Part model, mm, in its own coordinate system. A direction names the side the tool comes from. Give positions to 0.01 mm unless a question says otherwise; leave off trailing zeros. Loops run counter-clockwise (first coordinate to the right, second up) from the corner with the lowest first, then second, coordinate; pieces in that order, holes last. Notation, with made-up numbers: M 64,28.5 L 120,28.5 A29 cw 120,54.5 Z; hole C -7,29 d4. An arc over 180 degrees is marked long. Answer in a Markdown table with one row per item.
from build123d import *

# Parameters (mm, degrees)
SKETCH_1_W               = 58
SKETCH_1_H               = 44
SKETCH_1_R               = 1.6
EXTRUDE_1_DEPTH          = 1
SKETCH_2_W               = 132.5
SKETCH_2_H               = 90
EXTRUDE_2_DEPTH          = 1
SKETCH_6_W               = 15
SKETCH_6_H               = 90
CUT_EXTRUDE_4_DEPTH      = 1
CUT_EXTRUDE_4_DEPTH_BACK = 2
CUT_EXTRUDE_6_DEPTH      = 2
EXTRUDE_3_DEPTH          = 1
EXTRUDE_4_DEPTH          = 1
SKETCH_11_R              = 1.6
CUT_EXTRUDE_7_DEPTH      = 2
CUT_EXTRUDE_8_DEPTH      = 2
FILLET_3_R               = 2
SKETCH_14_R              = 1.6
CUT_EXTRUDE_9_DEPTH      = 2
SKETCH_15_R              = 9
CUT_EXTRUDE_10_DEPTH     = 2
CUT_EXTRUDE_11_DEPTH     = 2


with BuildPart() as part:
    # 草图1 → 凸台-拉伸1 (new body)
    with BuildSketch(Plane(origin=(0, 0, 0), x_dir=(0, 0, -1), z_dir=(1, 0, 0))):
        with Locations((19, -14.5)):
            Rectangle(SKETCH_1_W, SKETCH_1_H)
        Circle(SKETCH_1_R, mode=Mode.SUBTRACT)
        with Locations((17, 0)):
            Circle(SKETCH_1_R, mode=Mode.SUBTRACT)
        with Locations((0, -30.5)):
            Circle(SKETCH_1_R, mode=Mode.SUBTRACT)
        with Locations((17, -30.5)):
            Circle(SKETCH_1_R, mode=Mode.SUBTRACT)
        with Locations((31.5, -30.5)):
            Circle(SKETCH_1_R, mode=Mode.SUBTRACT)
    extrude(amount=EXTRUDE_1_DEPTH)

    # 草图2 → 凸台-拉伸2 (add)
    with BuildSketch(Plane(origin=(1, 0, 0), x_dir=(0, 0, -1), z_dir=(1, 0, 0))):
        with Locations((-18.25, 52.5)):
            Rectangle(SKETCH_2_W, SKETCH_2_H)
    extrude(amount=-EXTRUDE_2_DEPTH)

    # 草图6 → 切除-拉伸4 (cut, two sides)
    with BuildSketch(Plane(origin=(1, 0, 0), x_dir=(0, 0, -1), z_dir=(1, 0, 0))) as cut_extrude_4_sk:
        with Locations((40.5, 52.5)):
            Rectangle(SKETCH_6_W, SKETCH_6_H)
    extrude(amount=CUT_EXTRUDE_4_DEPTH, mode=Mode.SUBTRACT)
    extrude(cut_extrude_4_sk.sketch, amount=-CUT_EXTRUDE_4_DEPTH_BACK, mode=Mode.SUBTRACT)

    # 草图8 → 切除-拉伸6 (cut, through all)
    with BuildSketch(Plane(origin=(1, 0, 0), x_dir=(0, 0, -1), z_dir=(1, 0, 0))):
        Polygon((-84.5, 7.5), (-10, 7.5), (-10, 6.5), (48, 6.5), (48, 7.5), (33, 7.5), (33, 97.5), (-84.5, 97.5), align=None)
    extrude(amount=-CUT_EXTRUDE_6_DEPTH, mode=Mode.SUBTRACT)

    # 草图9 → 凸台-拉伸3 (add)
    with BuildSketch(Plane(origin=(1, 0, 0), x_dir=(0, 0, -1), z_dir=(1, 0, 0))):
        Polygon((-10, -32.5), (-10, 3.4), (-85.916522377, 1.4), (-95, -32.5), (-10, -36.5), align=None)
    extrude(amount=-EXTRUDE_3_DEPTH)

    # 草图10 → 凸台-拉伸4 (add)
    with BuildSketch(Plane(origin=(1, 0, 0), x_dir=(0, 0, -1), z_dir=(1, 0, 0))):
        Polygon((40.4, -45.5), (58.4, -45.5), (58.4, 6.5), (48, 6.5), (48, -36.5), (40.4, -36.5), align=None)
    extrude(amount=-EXTRUDE_4_DEPTH)

    # 草图11 → 切除-拉伸7 (cut, through all)
    with BuildSketch(Plane(origin=(1, 0, 0), x_dir=(0, 0, -1), z_dir=(1, 0, 0))):
        with Locations((45.4, -42.5)):
            Circle(SKETCH_11_R)
        with Locations((53.4, -42.5)):
            Circle(SKETCH_11_R)
    extrude(amount=-CUT_EXTRUDE_7_DEPTH, mode=Mode.SUBTRACT)

    # 草图13 → 切除-拉伸8 (cut, through all)
    with BuildSketch(Plane(origin=(1, 0, 0), x_dir=(0, 0, -1), z_dir=(1, 0, 0))):
        Polygon((24.2, 6.5), (58.4, -19.5), (58.4, 6.5), align=None)
    extrude(amount=-CUT_EXTRUDE_8_DEPTH, mode=Mode.SUBTRACT)

    # 圆角3
    fillet_3_edges = [part.edges().sort_by_distance(p)[0] for p in [
        (0.5, -32.5, 95),
        (0.5, 1.4, 85.916522377),
        (0.5, -45.5, -58.4),
        (0.5, -45.5, -40.4),
        (0.5, -36.5, -40.4),
        (0.5, 6.5, -24.2),
        (0.5, -19.5, -58.4),
    ]]
    fillet(fillet_3_edges, radius=FILLET_3_R)

    # 草图14 → 切除-拉伸9 (cut, through all)
    with BuildSketch(Plane(origin=(1, 0, 0), x_dir=(0, 0, -1), z_dir=(1, 0, 0))):
        with Locations((55.5, -30.5)):
            Circle(SKETCH_14_R)
    extrude(amount=-CUT_EXTRUDE_9_DEPTH, mode=Mode.SUBTRACT)

    # 草图15 → 切除-拉伸10 (cut, through all)
    with BuildSketch(Plane.ZY):
        with Locations((32, -16.5)):
            Circle(SKETCH_15_R)
    extrude(amount=-CUT_EXTRUDE_10_DEPTH, mode=Mode.SUBTRACT)

    # 草图16 → 切除-拉伸11 (cut, through all)
    with BuildSketch(Plane.ZY):
        with BuildLine():
            Line((-40.126719129, -22.148481915), (-23.2419273, -8.772218258))
            ThreePointArc((-23.2419273, -8.772218258), (-21.129326296, -8.5393617), (-20, -10.339896982))
            Line((-20, -10.339896982), (-20, -24.5))
            ThreePointArc((-20, -24.5), (-20.878679656, -26.621320344), (-23, -27.5))
            Line((-23, -27.5), (-31.5, -27.5))
            Line((-31.5, -27.5), (-38.263828178, -27.5))
            ThreePointArc((-38.263828178, -27.5), (-41.09707316, -25.48626714), (-40.126719129, -22.148481915))
        make_face()
        with BuildLine():
            Line((-14, -6), (-14, -24.5))
            ThreePointArc((-14, -24.5), (-13.121320344, -26.621320344), (-11, -27.5))
            Line((-11, -27.5), (-6, -27.5))
            ThreePointArc((-6, -27.5), (-3.878679656, -26.621320344), (-3, -24.5))
            Line((-3, -24.5), (-3, -6))
            ThreePointArc((-3, -6), (-3.878679656, -3.878679656), (-6, -3))
            Line((-6, -3), (-11, -3))
            ThreePointArc((-11, -3), (-13.121320344, -3.878679656), (-14, -6))
        make_face()
    extrude(amount=-CUT_EXTRUDE_11_DEPTH, mode=Mode.SUBTRACT)


solid = part.part
(1) Drill centre lines: line 1 along Y through (x, z) = (0.55, 0); line 2 along Z through (x, y) = (0.9, -0.5); line 3 along Y through (x, z) = (0.5, -30.5). Where is each one in solid material? Low to high.
Recorded:
| item | result |
|---|---|
| line 1 | y = -36.5 to -32.1, -28.9 to -1.6, 1.6 to 6.5 |
| line 2 | z = -33.41 to -18.52, -15.48 to -1.52, 1.52 to 86.43 |
| line 3 | y = -36.5 to -31.75, -29.25 to -27.5, -14.52 to 1.71 |
(2) Saw through at A-A (z = 0). Write the cut outline in (x, y), plus the area to 3 significant figures.
Recorded:
| item | result |
|---|---|
| outline | M 0,-36.5 L 1,-36.5 L 1,-32.1 L 0,-32.1 Z; M 0,-28.9 L 1,-28.9 L 1,-1.6 L 0,-1.6 Z; M 0,1.6 L 1,1.6 L 1,6.5 L 0,6.5 Z |
| area | 36.6 mm^2 |
(3) Saw through at D-D (x = 0.8). Give the number of separate pieces and of enclosed holes in the cut face, plus the area to 3 significant figures.
Recorded:
| item | result |
|---|---|
| separate pieces | 1 |
| enclosed holes | 11 |
| area | 4,780 mm^2 |
(4) Pull direction Y, two halves, no side cores. Call faces 1 (the face through (1, -19, 19)), 2 (the face through (0.49, -0.97, 1.27)), 3 (the face through (0.507, -14.861, 90.274)): +Y half, -Y half, draft (parallel to the pull), parting line (faces both ways), or undercut.
Recorded:
| item | result |
|---|---|
| face 1 | draft |
| face 2 | undercut |
| face 3 | +Y half |
(5) Which spindle directions (+Z, -Z, +X, -X, +Y, -Y) get a long thin tool onto all of the face, cutting with end or side? Do faces 4 (the face through (0.49, -26.64, -3.9)), 5 (the face through (0.51, -34.53, 51.84)). Say none if no direction does.
Recorded:
| item | result |
|---|---|
| face 4 | +X, -X |
| face 5 | +Z, +X, -X, -Y |
(6) Pin check, flat tips, straight feed: pin 1 Ø0.5 at (x, y) = (0.5, -42) entering from +Z; pin 2 Ø0.5 at (x, y) = (0.5, -13.5) entering from +Z; pin 3 Ø0.5 at (x, y) = (0.5, 4) entering from +Z. Stop position of each tip, or through.
Recorded:
| item | result |
|---|---|
| pin 1 | stops at z = -40.4 |
| pin 2 | stops at z = 89.98 |
| pin 3 | stops at z = 10 |
(7) Saw through at B-B (y = -12). Write the cut outline in (x, z).
Recorded:
| item | result |
|---|---|
| outline | M 0,-48.53 L 1,-48.53 L 1,-27.32 L 0,-27.32 Z; M 0,-20 L 1,-20 L 1,-14 L 0,-14 Z; M 0,-3 L 1,-3 L 1,24.21 L 0,24.21 Z; M 0,39.79 L 1,39.79 L 1,89.51 L 0,89.51 Z |
(8) Saw through at C-C (z = 32). Write the cut outline in (x, y).
Recorded:
| item | result |
|---|---|
| outline | M 0,-35.46 L 1,-35.46 L 1,-25.5 L 0,-25.5 Z; M 0,-7.5 L 1,-7.5 L 1,2.82 L 0,2.82 Z |
